Work out the finished part from the listing and answer in its coordinate system (mm). Face numbers are marked on the shaded views. A direction names the side the tool comes from. Round coordinates to 2 decimals unless told otherwise and drop trailing zeros. Write each loop counter-clockwise with the first axis right and the second up, starting at its lowest first coordinate (ties: lowest second). Pieces come first, ordered by that corner, then holes. Notation, with made-up numbers: (32.25, 41) -> (68.25, 41) arc R17 ccw to (68.25, 55) -> close; hole circle Ø9 at (41.5, 37). An arc over 180 degrees is marked (long way). One line per item, written item: value.
```python
from build123d import *

# Parameters (mm, degrees)
SKETCH1_R  = 0.95
BODY_DEPTH = 9.65
LOCK_DEPTH = 1


with BuildPart() as part:
    # Sketch1 → Body (new body)
    with BuildSketch(Plane(origin=(0, 0, 0), x_dir=(1, 0, 0), z_dir=(0, 1, 0))):
        Circle(SKETCH1_R)
    extrude(amount=BODY_DEPTH)

    # Sketch2 → Lock (add)
    with BuildSketch(Plane(origin=(0, 9.65, 0), x_dir=(1, 0, 0), z_dir=(0, 1, 0))):
        with BuildLine():
            ThreePointArc((-0.807774721, -0.5), (-0.95, 0), (-0.807774721, 0.5))
            Line((-0.807774721, 0.5), (-1.9, 0.5))
            Line((-1.9, 0.5), (-1.9, -0.5))
            Line((-1.9, -0.5), (-0.807774721, -0.5))
        make_face()
        with BuildLine():
            Line((1.9, 0.5), (0.807774721, 0.5))
            ThreePointArc((0.807774721, 0.5), (0.91375215, 0.259917309), (0.95, 0))
            ThreePointArc((0.95, 0), (0.91375215, -0.259917309), (0.807774721, -0.5))
            Line((0.807774721, -0.5), (1.9, -0.5))
            Line((1.9, -0.5), (1.9, 0.5))
        make_face()
    extrude(amount=-LOCK_DEPTH)


solid = part.part
```
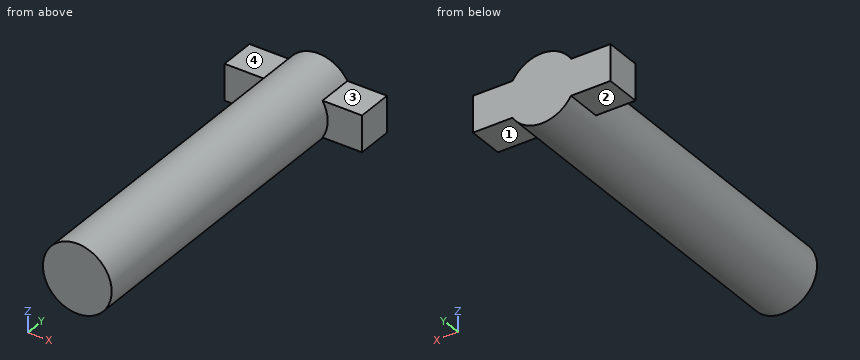
(1) Consider probe 1 along X at (y, z) = (7.5, 0.05); probe 2 along Z at (x, y) = (-0.5, 7). Determine where each line is inside the solid, lowest interval first.
Reported:
probe 1: x = -0.95 to 0.95
probe 2: z = -0.81 to 0.81
(2) Find section A-A on z = 0. Give the vertices of the cut face in (x, y), plus the area to 3 significant figures.
Reported:
outline: (-1.9, 8.65) -> (-0.95, 8.65) -> (-0.95, 0) -> (0.95, 0) -> (0.95, 8.65) -> (1.9, 8.65) -> (1.9, 9.65) -> (-1.9, 9.65) -> close
area: 20.2 mm2
(3) Flat-ended cylindrical pins translate along their axes: pin 1 Ø0.5 at (x, z) = (1.5, 0) entering from -Y; pin 2 Ø1.1 at (x, y) = (1, 9) entering from +Z; pin 3 Ø1.1 at (x, y) = (1.5, 9.5) entering from -Z. Find the tip coordinate at first contact, or state that the pin passes through.
Reported:
pin 1: stops at y = 8.65
pin 2: stops at z = 0.84
pin 3: stops at z = -0.5
(4) Find section D-D on z = 0.4. Give the vertices of the cut face in (x, y).
Reported:
outline: (-1.9, 8.65) -> (-0.86, 8.65) -> (-0.86, 0) -> (0.86, 0) -> (0.86, 8.65) -> (1.9, 8.65) -> (1.9, 9.65) -> (-1.9, 9.65) -> close
(5) Find section C-C on x = 1.35. Give the vertices of the cut face in (y, z).
Reported:
outline: (8.65, -0.5) -> (9.65, -0.5) -> (9.65, 0.5) -> (8.65, 0.5) -> close
(6) Find section B-B on y = 1.5. Give the vertices of the cut face in (x, z).
Reported:
outline: circle Ø1.9 at (0, 0)
(7) A tool of negligible diameter and unlimited length cuts with its end or side. For the marked faces 1, 2, 3 and 4, from which of +Z, -Z, +X, -X, +Y, -Y can it reach the whole face along a straight path? Write none if from no direction.
Reported:
face 1: -Z, +X, +Y, -Y
face 2: -Z, -X, +Y, -Y
face 3: +Z, +X, +Y, -Y
face 4: +Z, -X, +Y, -Y
